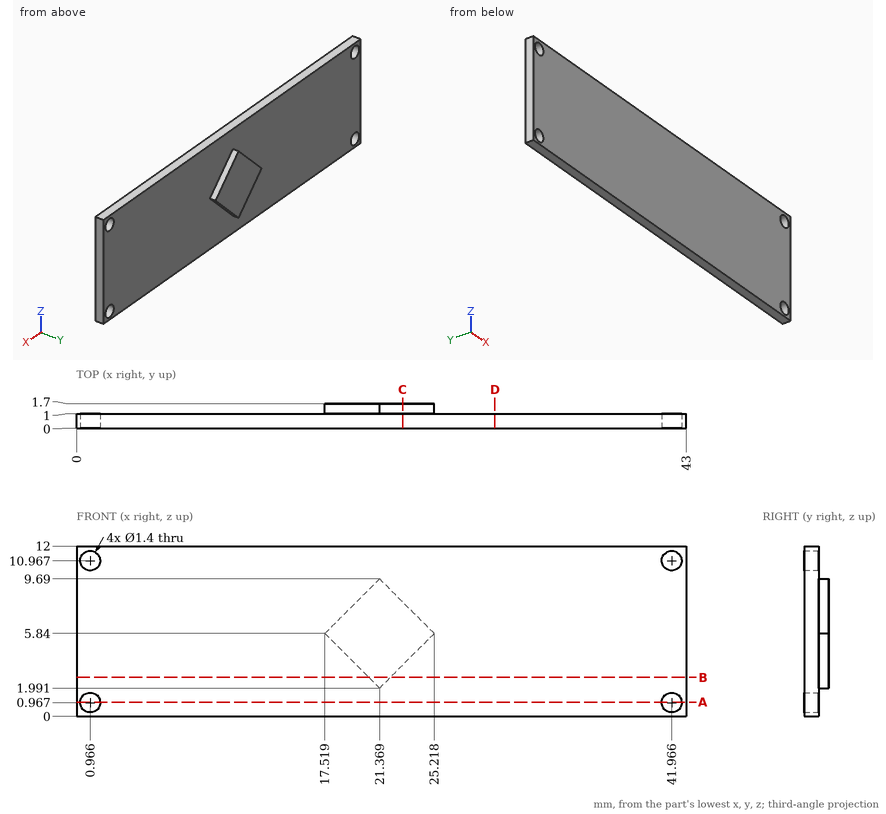
Design review of the part shown in the three views and the two pictorial views. Dimensions are in mm from the part's minimum x, y and z. Round coordinates to 2 decimals unless told otherwise and drop trailing zeros. Loops run counter-clockwise (first coordinate to the right, second up) from the corner with the lowest first, then second, coordinate; pieces in that order, holes last. Notation, with made-up numbers: M 35.5,10 L 92.5,10 A15 cw 92.5,18 Z; hole C -23.75,-21.5 d8. An arc over 180 degrees is marked long. Put each result on its own line as item: value.
Q1. To check wall thickness, follow L1, parallel to X at y = 0.45, z = 11.25 (1 decimal); L2, parallel to Y at x = 25, z = 4.25; L3, parallel to X at y = 1.65, z = 9. State the ranges of each line that lie inside material, in increasing order.
Result set:
L1: x = 0 to 0.3, 1.6 to 41.3, 42.6 to 43
L2: y = 0 to 1
L3: x = 20.68 to 22.06
Q2. Consider section A-A, the plane z = 1. Count the separate pieces of the cut face and the enclosed holes in it.
Result set:
separate pieces: 3
enclosed holes: 0
Q3. Consider section D-D, the plane x = 29.5. Give the boundary of the cut face in (y, z), then the cut area to 3 significant figures.
Result set:
outline: M 0,0 L 1,0 L 1,12 L 0,12 Z
area: 12.0 mm²
Q4. Consider section C-C, the plane x = 23. Give the boundary of the cut face in (y, z).
Result set:
outline: M 0,0 L 1,0 L 1,3.62 L 1.7,3.62 L 1.7,8.06 L 1,8.06 L 1,12 L 0,12 Z
Q5. For pin 1 (2 mm diameter, centred on x = 0.97, z = 0.97, fed in from +Y); pin 2 (1 mm diameter, centred on x = 13, z = 5, fed in from -Y); pin 3 (1.3 mm diameter, centred on x = 41.97, z = 10.97, fed in from -Y), all flat-tipped, find the tip position at first contact; note any pin that passes through.
Result set:
pin 1: stops at y = 1
pin 2: stops at y = 0
pin 3: passes through
Q6. Consider section B-B, the plane z = 2.75. Give the boundary of the cut face in (x, y).
Result set:
outline: M 0,0 L 43,0 L 43,1 L 22.13,1 L 22.13,1.7 L 20.61,1.7 L 20.61,1 L 0,1 Z
